from build123d import *

# Parameters (mm, degrees)
F0_W     = 46
F0_H     = 2
F0_R     = 1.5
F0_R_2   = 0.575
F0_H_2   = 21
F0_R_3   = 8.1
F1_DEPTH = 2
F2_DEPTH = 25
F3_DEPTH = 7
F4_DEPTH = 12
F5_R     = 2
F7_DEPTH = 52


with BuildPart() as f1:
    # F0 (on Top) → F1 (new body)
    with BuildSketch(Plane.XY):
        with Locations((1.93201, 4.360505)):
            Rectangle(F0_W, F0_H)
        with Locations((-19.06799, 1.360505)):
            Circle(F0_R)
        with Locations((-19.06799, 1.360505)):
            Circle(F0_R_2, mode=Mode.SUBTRACT)
        with Locations((22.93201, -15.639495)):
            Circle(F0_R)
        with Locations((22.93201, -15.639495)):
            Circle(F0_R_2, mode=Mode.SUBTRACT)
        with Locations((22.93201, 1.360505)):
            Circle(F0_R)
        with Locations((22.93201, 1.360505)):
            Circle(F0_R_2, mode=Mode.SUBTRACT)
        with Locations((-19.06799, -15.639495)):
            Circle(F0_R)
        with Locations((-19.06799, -15.639495)):
            Circle(F0_R_2, mode=Mode.SUBTRACT)
        with Locations((1.93201, -7.139495)):
            Rectangle(F0_W, F0_H_2)
        with Locations((-19.06799, -15.639495)):
            Circle(F0_R, mode=Mode.SUBTRACT)
        with Locations((22.93201, -15.639495)):
            Circle(F0_R, mode=Mode.SUBTRACT)
        with Locations((-11.06799, -7.139495)):
            Circle(F0_R_3, mode=Mode.SUBTRACT)
        with Locations((-19.06799, 1.360505)):
            Circle(F0_R, mode=Mode.SUBTRACT)
        with Locations((14.93201, -7.139495)):
            Circle(F0_R_3, mode=Mode.SUBTRACT)
        with Locations((22.93201, 1.360505)):
            Circle(F0_R, mode=Mode.SUBTRACT)
        Polygon((-21.06799, 5.360505), (-23.06799, 5.360505), (-23.06799, -19.639495), (-21.06799, -19.639495), (-21.06799, -17.639495), (-21.06799, 3.360505), align=None)
        Polygon((-21.06799, -17.639495), (-21.06799, -19.639495), (26.93201, -19.639495), (26.93201, -17.639495), (24.93201, -17.639495), align=None)
        Polygon((26.93201, 5.360505), (24.93201, 5.360505), (24.93201, 3.360505), (24.93201, -17.639495), (26.93201, -17.639495), align=None)
    extrude(amount=F1_DEPTH)

    # F0 (on Top) → F2 (join)
    with BuildSketch(Plane.XY):
        Polygon((-21.06799, 5.360505), (-23.06799, 5.360505), (-23.06799, -19.639495), (-21.06799, -19.639495), (-21.06799, -17.639495), (-21.06799, 3.360505), align=None)
        with Locations((1.93201, 4.360505)):
            Rectangle(F0_W, F0_H)
        Polygon((-21.06799, -17.639495), (-21.06799, -19.639495), (26.93201, -19.639495), (26.93201, -17.639495), (24.93201, -17.639495), align=None)
        Polygon((26.93201, 5.360505), (24.93201, 5.360505), (24.93201, 3.360505), (24.93201, -17.639495), (26.93201, -17.639495), align=None)
        Polygon((-21.06799, -19.639495), (-23.06799, -19.639495), (-23.06799, -29.639495), (26.93201, -29.639495), (26.93201, -19.639495), align=None)
    extrude(amount=F2_DEPTH)

    # F0 (on Top) → F3 (join)
    with BuildSketch(Plane.XY):
        with Locations((-19.06799, 1.360505)):
            Circle(F0_R)
        with Locations((-19.06799, 1.360505)):
            Circle(F0_R_2, mode=Mode.SUBTRACT)
        with Locations((-19.06799, -15.639495)):
            Circle(F0_R)
        with Locations((-19.06799, -15.639495)):
            Circle(F0_R_2, mode=Mode.SUBTRACT)
        with Locations((22.93201, 1.360505)):
            Circle(F0_R)
        with Locations((22.93201, 1.360505)):
            Circle(F0_R_2, mode=Mode.SUBTRACT)
        with Locations((22.93201, -15.639495)):
            Circle(F0_R)
        with Locations((22.93201, -15.639495)):
            Circle(F0_R_2, mode=Mode.SUBTRACT)
    extrude(amount=F3_DEPTH)

    # F0 (on Top) → F4 (join)
    with BuildSketch(Plane.XY):
        with Locations((-19.06799, 1.360505)):
            Circle(F0_R_2)
        with Locations((-19.06799, -15.639495)):
            Circle(F0_R_2)
        with Locations((22.93201, -15.639495)):
            Circle(F0_R_2)
        with Locations((22.93201, 1.360505)):
            Circle(F0_R_2)
    extrude(amount=F4_DEPTH)

    # F5
    f5_edges = [f1.edges().sort_by_distance(p)[0] for p in [
        (1.93201, 5.360505, 0),
        (26.93201, 5.360505, 12.5),
        (-23.06799, 5.360505, 12.5),
    ]]
    fillet(f5_edges, radius=F5_R)

    # F6 (on face) → F7 (cut)
    with BuildSketch(Plane.YZ.offset(26.93201)):
        Polygon((-29.639495, 0), (-21.639495, 25), (-29.639495, 25), align=None)
    extrude(amount=-F7_DEPTH, mode=Mode.SUBTRACT)


solid = f1.part
Work out the finished part from the listing and answer in its coordinate system (mm). A direction names the side the tool comes from. Round coordinates to 2 decimals unless told otherwise and drop trailing zeros. Write each loop counter-clockwise with the first axis right and the second up, starting at its lowest first coordinate (ties: lowest second). Pieces come first, ordered by that corner, then holes.
1) A cutting plane is placed at C-C (x = 7.5). Give the vertices of the cut face in (y, z), plus the area to 3 significant figures.
2) Given pin 1 Ø1.5 at (x, y) = (-19.5, -15.5) entering from +Z; pin 2 Ø8 at (x, z) = (-12, 15.5) entering from -Y; pin 3 Ø1 at (x, z) = (13.5, 19) entering from -Y, each flat-ended and moving along its own axis, determine where each tip first touches the part or whether it passes through.
3) Straight lines are drawn through the part: line 1 (X direction, y = 1.5, z = 4.5); line 2 (X direction, y = -1, z = 11); line 3 (Y direction, x = -18, z = 5.5). For each, find the intervals that lie inside material, in ascending order.
4) A cutting plane is placed at B-B (y = -4). Give the vertices of the cut face in (x, z), plus the area to 3 significant figures.
5) A tool of negligible diameter and unlimited length cuts with its end or side. For faces 1 (the flat face through (24, -16, 7)), 2 (the flat face through (2.282, -25.695, 12.325)), from which of +Z, -Z, +X, -X, +Y, -Y can it reach the whole face along a straight path? Write none if from no direction.
6) A cutting plane is placed at D-D (z = 20). Give the vertices of the cut face in (x, y), plus the area to 3 significant figures.
7) A cutting plane is placed at A-A (z = 8). Give the number of separate pieces and of enclosed holes in the cut face, plus the area to 3 significant figures.
Completed:
1. outline: (-29.64, 0) - (-10.36, 0) - (-10.36, 2) - (-17.64, 2) - (-17.64, 25) - (-21.64, 25) - close; (-3.92, 0) - (3.36, 0) arc R2 ccw to (5.36, 2) - (5.36, 25) - (3.36, 25) - (3.36, 2) - (-3.92, 2) - close
1. area: 278 mm2
2. pin 1: stops at z = 12
2. pin 2: stops at y = -25.96
2. pin 3: stops at y = -23.72
3. line 1: x = -23.07 to -21.07, -20.56 to -17.57, 21.44 to 24.43, 24.93 to 26.93
3. line 2: x = -23.07 to -21.07, 24.93 to 26.93
3. line 3: y = -27.88 to -17.64, -16.69 to -14.59, 0.31 to 2.41, 3.36 to 5.36
4. outline: (-23.07, 0) - (-18.53, 0) - (-18.53, 2) - (-21.07, 2) - (-21.07, 25) - (-23.07, 25) - close; (-3.6, 0) - (7.47, 0) - (7.47, 2) - (-3.6, 2) - close; (22.4, 0) - (26.93, 0) - (26.93, 25) - (24.93, 25) - (24.93, 2) - (22.4, 2) - close
4. area: 132 mm2
5. face 1: +Z
5. face 2: +Z, +X, -X, -Y
6. outline: (-23.07, -23.24) - (26.93, -23.24) - (26.93, 3.36) arc R2 ccw to (24.93, 5.36) - (-21.07, 5.36) arc R2 ccw to (-23.07, 3.36) - close; hole (-21.07, -17.64) - (24.93, -17.64) - (24.93, 3.36) - (-21.07, 3.36) - close
6. area: 462 mm2
7. separate pieces: 5
7. enclosed holes: 1
7. area: 658 mm2
